```python
from build123d import *

# Parameters (mm, degrees)
SKETCH4_R          = 9.0551
SKETCH4_R_2        = 8.89635
CUT_EXTRUDE2_DEPTH = 7.112
CUT_EXTRUDE1_DEPTH = 7.112
CIRPATTERN1_COUNT  = 28
SKETCH6_R          = 8.7376
CUT_EXTRUDE3_DEPTH = 6.35


with BuildPart() as part:
    # Sketch1 → Revolve1 (revolve)
    with BuildSketch(Plane.XY, mode=Mode.PRIVATE) as revolve1_sk:
        with BuildLine():
            Line((-8.7376, 3.175), (8.7376, 3.175))
            Line((8.7376, 3.175), (8.7376, 11.176))
            Line((8.7376, 11.176), (7.7343, 11.176))
            ThreePointArc((7.7343, 11.176), (7.003726949, 10.549537058), (6.731, 9.6266))
            Line((6.731, 9.6266), (6.731, 9.0551))
            Line((6.731, 9.0551), (-0.381, 9.0551))
            Line((-0.381, 9.0551), (-0.381, 9.6266))
            ThreePointArc((-0.381, 9.6266), (-0.653726949, 10.549537058), (-1.3843, 11.176))
            Line((-1.3843, 11.176), (-2.3876, 11.176))
            Line((-2.3876, 11.176), (-2.3876, 8.7376))
            Line((-2.3876, 8.7376), (-8.7376, 8.7376))
            Line((-8.7376, 8.7376), (-8.7376, 3.175))
        make_face()
    revolve(revolve1_sk.sketch.rotate(Axis((-8.7376, 0, 0), (1, 0, 0)), 90), axis=Axis((-8.7376, 0, 0), (1, 0, 0)))

    # Sketch4 → Cut-Extrude2 (cut)
    with BuildSketch(Plane(origin=(-0.381, 0, 0), x_dir=(0, 0, -1), z_dir=(1, 0, 0))):
        Circle(SKETCH4_R)
        Circle(SKETCH4_R_2, mode=Mode.SUBTRACT)
    extrude(amount=CUT_EXTRUDE2_DEPTH, mode=Mode.SUBTRACT)

    # Sketch3 → Cut-Extrude1 (cut)
    with BuildSketch(Plane(origin=(-0.381, 0, 0), x_dir=(0, 0, -1), z_dir=(1, 0, 0))):
        with BuildLine():
            Line((-0.643388094, 8.873054439), (-0.340062676, 8.222570981))
            Line((-0.340062676, 8.222570981), (0.340062676, 8.222570981))
            Line((0.340062676, 8.222570981), (0.643388094, 8.873054439))
            ThreePointArc((0.643388094, 8.873054439), (0, 8.89635), (-0.643388094, 8.873054439))
        make_face()
    cut_extrude1 = extrude(amount=CUT_EXTRUDE1_DEPTH, mode=Mode.SUBTRACT)

    # CirPattern1: Cut-Extrude1 ×28 about axis
    cirpattern1_axis = Axis((0, 0, 0), (1, 0, 0))
    for i in range(1, CIRPATTERN1_COUNT):
        add(cut_extrude1.rotate(cirpattern1_axis, i * 360 / CIRPATTERN1_COUNT), mode=Mode.SUBTRACT)

    # Sketch6 → Cut-Extrude3 (cut)
    with BuildSketch(Plane.ZY.offset(8.7376)):
        Circle(SKETCH6_R)
    extrude(amount=-CUT_EXTRUDE3_DEPTH, mode=Mode.SUBTRACT)


solid = part.part
```
Verification items for the finished model (mm, model axes). A direction names the side the tool comes from. Give positions to 0.01 mm unless a question says otherwise; leave off trailing zeros. Loops run counter-clockwise (first coordinate to the right, second up) from the corner with the lowest first, then second, coordinate; pieces in that order, holes last. Notation, with made-up numbers: M 30.25,59 L 59.25,59 A12 ccw 59.25,72 Z; hole C -12.75,12.25 d5. An arc over 180 degrees is marked long. One line per question, with ' | ' between items.
Item 1: Section check C-C, the plane x = -0.75. Record the cut outline in (y, z) (3 decimals), plus the area to 3 significant figures.
Completed:
outline: C 0,0 d21.367; hole C 0,0 d6.35 | area: 327 mm^2
Item 2: Section check A-A, the plane z = 0. Record the cut outline in (x, y) (3 decimals).
Completed:
outline: M -2.388,-11.176 L -1.384,-11.176 A1.698 ccw -0.381,-9.627 L -0.381,-8.223 L 6.731,-8.223 L 6.731,-9.627 A1.698 ccw 7.734,-11.176 L 8.738,-11.176 L 8.738,-3.175 L -2.388,-3.175 Z; M -2.388,3.175 L 8.738,3.175 L 8.738,11.176 L 7.734,11.176 A1.698 ccw 6.731,9.627 L 6.731,8.223 L -0.381,8.223 L -0.381,9.627 A1.698 ccw -1.384,11.176 L -2.388,11.176 Z
Item 3: Tool access check on faces 4 (the face through (8.738, -3, -2)), 5 (the face through (6.731, 0, 9)). Record the directions out of +Z, -Z, +X, -X, +Y, -Y that give a thin tool (end or side, any length) a straight path to the whole face; none if there is none.
Completed:
face 4: +Z, -Z, +X, +Y, -Y | face 5: none
Item 4: Draft check along Z on faces 1 (the face through (-1.89, 6.8, -8.87)), 2 (the face through (3.25, 1.93, -2.52)), 3 (the face through (-2.388, 3, 2)). Enter one of: +Z half, -Z half, draft (parallel to the pull), parting line (faces both ways), or undercut.
Completed:
face 1: parting line | face 2: undercut | face 3: draft
Item 5: Thickness scan on line 1 (X direction, y = -5.25, z = -7); line 2 (Y direction, x = 4.25, z = 0) (3 decimals); line 3 (Y direction, x = -2, z = 0) (3 decimals). Record the ranges inside material, lowest first. Write a range as [from, to].
Completed:
line 1: x = [-2.39, -0.38], [6.73, 8.74] | line 2: y = [-8.223, -3.175], [3.175, 8.223] | line 3: y = [-11.176, -3.175], [3.175, 11.176]
Item 6: Depth check by flat-ended pin: P1, Ø6, axis at x = 4, z = -1, coming from the -Y side; P2, Ø0.5, axis at x = 4, z = 0, coming from the -Y side; P3, Ø3, axis at x = 0.5, z = 4.5, coming from the +Y side; P4, Ø10, axis at y = -0.5, z = 1, coming from the +X side. Enter the tip coordinate at first touch or a pass-through.
Completed:
P1: stops at y = -10.5 | P2: stops at y = -8.22 | P3: stops at y = 10.1 | P4: stops at x = 8.74
